Check sheet for the modelled part. Datum: model origin and axes. Units: mm. A direction names the side the tool comes from. Coordinates: 2 decimals unless noted, no trailing zeros. Loops run counter-clockwise (first coordinate to the right, second up) from the corner with the lowest first, then second, coordinate; pieces in that order, holes last. Notation, with made-up numbers: M 65,-16 L 89,-16 A37 ccw 89,22 Z; hole C -7,69.5 d7. An arc over 180 degrees is marked long. Return JSON: item names as keys, results as strings.
from build123d import *

# Parameters (mm, degrees)
SKETCH1_R             = 2.25
SKETCH1_R_2           = 1.5
BOSS_EXTRUDE1_DEPTH   = 3
CORTAR_EXTRUIR1_REACH = 34.469
CROQUIS1_W            = 32.5
CROQUIS1_H            = 7.5


with BuildPart() as part:
    # Sketch1 → Boss-Extrude1 (new body)
    with BuildSketch(Plane.XY):
        with BuildLine():
            Line((-13.25, 27.95), (13.25, 27.95))
            ThreePointArc((13.25, 27.95), (15.371320344, 27.071320344), (16.25, 24.95))
            Line((16.25, 24.95), (16.25, -24.95))
            ThreePointArc((16.25, -24.95), (15.371320344, -27.071320344), (13.25, -27.95))
            Line((13.25, -27.95), (-13.25, -27.95))
            ThreePointArc((-13.25, -27.95), (-15.371320344, -27.071320344), (-16.25, -24.95))
            Line((-16.25, -24.95), (-16.25, 24.95))
            ThreePointArc((-16.25, 24.95), (-15.371320344, 27.071320344), (-13.25, 27.95))
        make_face()
        with Locations((-5, 24.45)):
            Circle(SKETCH1_R, mode=Mode.SUBTRACT)
        with Locations((5, 24.45)):
            Circle(SKETCH1_R_2, mode=Mode.SUBTRACT)
        with Locations(Location((5, -24.45, 0), (0, 0, 180))):
            Circle(SKETCH1_R_2, mode=Mode.SUBTRACT)
        with Locations(Location((-5, -24.45, 0), (0, 0, 180))):
            Circle(SKETCH1_R, mode=Mode.SUBTRACT)
        Polygon((-10.25, 20.45), (10.25, 20.45), (10.25, 15.45), (13.25, 15.45), (13.25, 10.45), (10.25, 10.45), (10.25, 5.45), (13.25, 5.45), (13.25, 0.45), (10.25, 0.45), (10.25, -20.45), (-10.25, -20.45), (-10.25, 0.45), (-13.25, 0.45), (-13.25, 5.45), (-10.25, 5.45), (-10.25, 10.45), (-13.25, 10.45), (-13.25, 15.45), (-10.25, 15.45), align=None, mode=Mode.SUBTRACT)
    extrude(amount=BOSS_EXTRUDE1_DEPTH)

    # Croquis1 → Cortar-Extruir1 (cut, up to next)
    with BuildSketch(Plane.XY.offset(3), mode=Mode.PRIVATE) as cortar_extruir1_sk1:
        with Locations((0, -24.2)):
            Rectangle(CROQUIS1_W, CROQUIS1_H)
    cortar_extruir1_tool1 = extrude(cortar_extruir1_sk1.sketch, amount=-CORTAR_EXTRUIR1_REACH, mode=Mode.PRIVATE) & part.part
    add(cortar_extruir1_tool1.solids().sort_by_distance((0, -24.2, 3))[0], mode=Mode.SUBTRACT)


solid = part.part
1) Section check C-C on y = 24.45. Record the cut outline in (x, z).
Answers:
{"outline": "M -16.25,0 L -7.25,0 L -7.25,3 L -16.25,3 Z; M -2.75,0 L 3.5,0 L 3.5,3 L -2.75,3 Z; M 6.5,0 L 16.25,0 L 16.25,3 L 6.5,3 Z"}
2) Draft check along X on faces 4 (the face through (-16.25, 2, 1)), 5 (the face through (-12, 15.45, 1)), 6 (the face through (-13, -20.45, 2)). Enter one of: +X half, -X half, draft (parallel to the pull), parting line (faces both ways), or undercut.
Answers:
{"face 4": "-X half", "face 5": "undercut", "face 6": "draft"}
3) Section check B-B on x = 5. Record the cut outline in (y, z), then the cut area to 3 significant figures.
Answers:
{"outline": "M 20.45,0 L 22.95,0 L 22.95,3 L 20.45,3 Z; M 25.95,0 L 27.95,0 L 27.95,3 L 25.95,3 Z", "area": "13.5 mm²"}
4) Section check D-D on x = 12. Record the cut outline in (y, z).
Answers:
{"outline": "M -20.45,0 L 0.45,0 L 0.45,3 L -20.45,3 Z; M 5.45,0 L 10.45,0 L 10.45,3 L 5.45,3 Z; M 15.45,0 L 27.95,0 L 27.95,3 L 15.45,3 Z"}
5) Scan lines: line 1 along X through (y, z) = (-15.5, 2); line 2 along X through (y, z) = (3.5, 1.75); line 3 along Y through (x, z) = (5, 1.35). Record each from-to range of solid material in increasing order. Write a range as [from, to].
Answers:
{"line 1": "[-16.25, -10.25], [10.25, 16.25]", "line 2": "[-16.25, -13.25], [13.25, 16.25]", "line 3": "[20.45, 22.95], [25.95, 27.95]"}
6) Section check A-A on y = -4. Record the cut outline in (x, z).
Answers:
{"outline": "M -16.25,0 L -10.25,0 L -10.25,3 L -16.25,3 Z; M 10.25,0 L 16.25,0 L 16.25,3 L 10.25,3 Z"}
7) Set-up check for faces 1 (the face through (-12, 10.45, 1)), 2 (the face through (11, 9, 3)), 3 (the face through (-10.25, 18, 1)): record each of +Z, -Z, +X, -X, +Y, -Y from which the full face is reachable in a straight line by a thin tool's end or side.
Answers:
{"face 1": "+Z, -Z", "face 2": "+Z, +X, -X, +Y, -Y", "face 3": "+Z, -Z, -Y"}
